Study the drawing (mm; zero at the part's minimum x, y, z) and answer. A direction names the side the tool comes from. Coordinates: 2 decimals unless noted, no trailing zeros. Order: outer loops, then holes, each group sorted by start corner. A loop starts at its lowest first (then second) coordinate and runs counter-clockwise, first axis right, second up.
1. Determine the mould class of the marked faces 3, 4, 5 and 6 for opening direction Y: +Y half, -Y half, draft (parallel to the pull), parting line (faces both ways), or undercut.
2. A tool of negligible diameter and unlimited length cuts with its end or side. For the marked faces 1 and 2, from which of +Z, -Z, +X, -X, +Y, -Y can it reach the whole face along a straight path? Write none if from no direction.
3. The part is cut by section C-C, the plane x = 69. Give the vertices of the cut face in (y, z).
4. The part is cut by section B-B, the plane y = 21. Give the vertices of the cut face in (x, z) (3 decimals).
5. Find the intervals of material crossed by probe 1 along Y at (x, z) = (66, 6.5); probe 2 along X at (y, z) = (21, 1.5) (3 decimals); probe 3 along X at (y, z) = (27, 19) (1 decimal), in increasing order.
6. The part is cut by section D-D, the plane y = 35.5. Give the vertices of the cut face in (x, z), then the cut area to 3 significant figures.
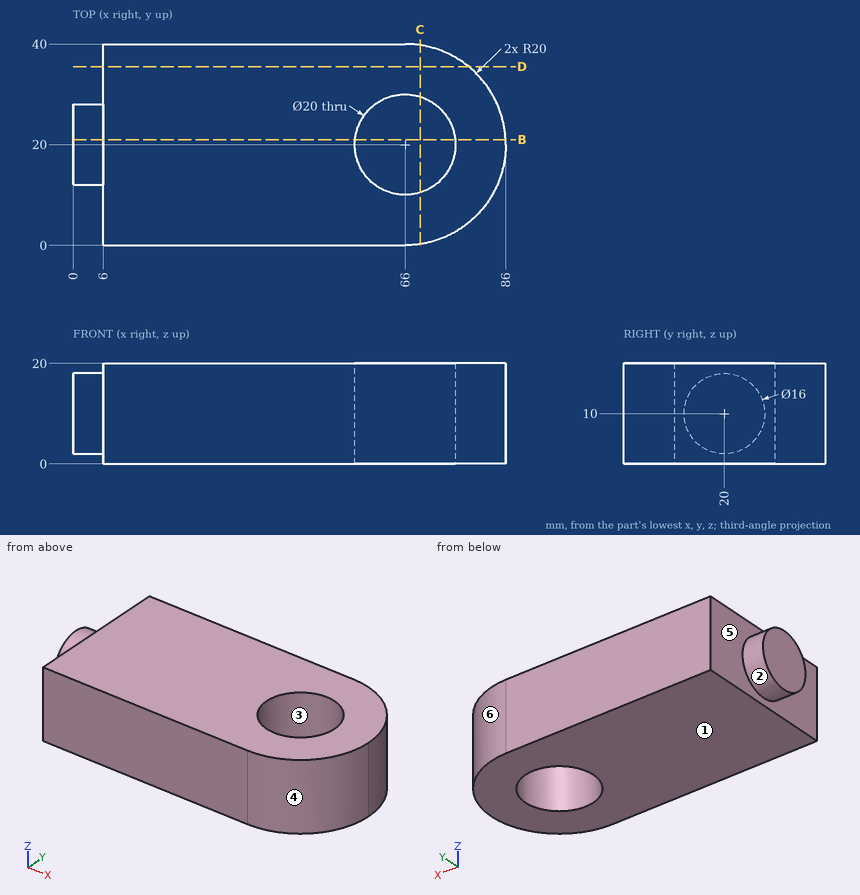
Geometry says:
1. face 3: undercut
1. face 4: -Y half
1. face 5: draft
1. face 6: +Y half
2. face 1: -Z, +X, -X, +Y, -Y
2. face 2: -X
3. outline: (0.23, 0) - (10.46, 0) - (10.46, 20) - (0.23, 20) - close; (29.54, 0) - (39.77, 0) - (39.77, 20) - (29.54, 20) - close
4. outline: (0, 2.063) - (6, 2.063) - (6, 0) - (56.05, 0) - (56.05, 20) - (6, 20) - (6, 17.937) - (0, 17.937) - close; (75.95, 0) - (85.975, 0) - (85.975, 20) - (75.95, 20) - close
5. probe 1: y = 0 to 10, 30 to 40
5. probe 2: x = 6 to 56.05, 75.95 to 85.975
5. probe 3: x = 6 to 58.9, 73.1 to 84.7
6. outline: (6, 0) - (78.64, 0) - (78.64, 20) - (6, 20) - close
6. area: 1,450 mm2
